from build123d import *

# Parameters (mm, degrees)
F0_W     = 38.1
F0_H     = 63.5
F1_DEPTH = 9.525
F2_W     = 38.1
F2_H     = 9.525
F3_DEPTH = 31.75
F4_R     = 8.75
F5_DEPTH = 6.35
F6_R     = 6.35
F7_DEPTH = 25.4
F4_R_2   = 8.7503
F8_DEPTH = 6.35


with BuildPart() as f1:
    # F0 (on Top) → F1 (new body)
    with BuildSketch(Plane.XY):
        with Locations((19.05, 31.75)):
            Rectangle(F0_W, F0_H)
    extrude(amount=F1_DEPTH)

    # F2 (on face) → F3 (join)
    with BuildSketch(Plane.XY.offset(9.525)):
        with Locations((19.05, 4.7625)):
            Rectangle(F2_W, F2_H)
    extrude(amount=F3_DEPTH)

    # F4 (on face) → F5 (cut)
    with BuildSketch(Plane(origin=(0, 0, 0), x_dir=(1, 0, 0), z_dir=(0, 0, -1))):
        with Locations((19.05, -44.45)):
            Circle(F4_R)
    extrude(amount=-F5_DEPTH, mode=Mode.SUBTRACT)

    # F6 (on face) → F7 (cut)
    with BuildSketch(Plane(origin=(0, 9.525, 0), x_dir=(-1, 0, 0), z_dir=(0, 1, 0))):
        with Locations((-19.05, 28.575)):
            Circle(F6_R)
    extrude(amount=-F7_DEPTH, mode=Mode.SUBTRACT)

    # F4 (on face) → F8 (cut)
    with BuildSketch(Plane(origin=(0, 0, 0), x_dir=(1, 0, 0), z_dir=(0, 0, -1))):
        with Locations((19.05, -44.45)):
            Circle(F4_R)
        with Locations((19.05, -12.7)):
            Circle(F4_R_2)
    extrude(amount=-F8_DEPTH, mode=Mode.SUBTRACT)


solid = f1.part
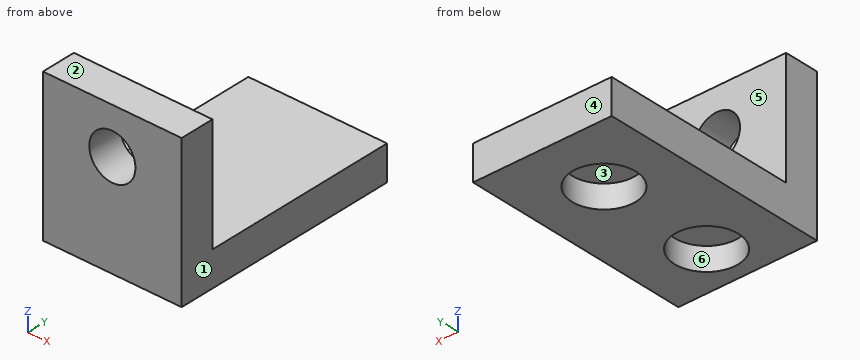
Check sheet for the modelled part. Datum: model origin and axes. Units: mm. Face numbers are marked on the shaded views. A direction names the side the tool comes from. Coordinates: 2 decimals unless noted, no trailing zeros. Loops run counter-clockwise (first coordinate to the right, second up) from the corner with the lowest first, then second, coordinate; pieces in that order, holes last. Notation, with made-up numbers: (40.5, 66.25) -> (65.5, 66.25) arc R14 ccw to (65.5, 70.25) -> close; hole circle Ø1 at (80.5, 73.25). An arc over 180 degrees is marked (long way). Write item = value, one per line. Start each with the question number.
1. Section check B-B on y = 44.45. Record the cut outline in (x, z) (3 decimals), then the cut area to 3 significant figures.
2. Section check D-D on z = 33.5. Record the cut outline in (x, y) (3 decimals).
3. Tool access check on the marked faces 4, 5 and 6. Record the directions out of +Z, -Z, +X, -X, +Y, -Y that give a thin tool (end or side, any length) a straight path to the whole face; none if there is none.
4. Section check A-A on x = 19.05. Record the cut outline in (y, z) (3 decimals), then the cut area to 3 significant figures.
5. Depth check by flat-ended pin: P1, Ø16, axis at x = 19.05, y = 12.7, coming from the -Z side; P2, Ø1, axis at x = 4.5, z = 28, coming from the -Y side; P3, Ø4, axis at x = 19.5, y = 19, coming from the +Z side (3 decimals); P4, Ø16, axis at x = 16.5, z = 27.5, coming from the +Y side (3 decimals). Enter the tip coordinate at first touch or a pass-through.
6. Material ranges on line 1 (Y direction, x = 19.05, z = 5); line 2 (Y direction, x = 2.5, z = 33.5) (3 decimals); line 3 (Z direction, x = 19, y = 2) (3 decimals), recorded low to high.
7. Section check C-C on y = 7.5. Record the cut outline in (x, z) (3 decimals).
8. Draft check along X on the marked faces 1, 2 and 3. Enter one of: released by +X, released by -X, zero draft, split by the parting line, or undercut.
Responses:
q1.outline = (0, 0) -> (10.3, 0) -> (10.3, 6.35) -> (27.8, 6.35) -> (27.8, 0) -> (38.1, 0) -> (38.1, 9.525) -> (0, 9.525) -> close
q1.area = 252 mm2
q2.outline = (0, 0) -> (15.042, 0) -> (15.042, 9.525) -> (0, 9.525) -> close; (23.058, 0) -> (38.1, 0) -> (38.1, 9.525) -> (23.058, 9.525) -> close
q3.face_4 = +Z, -Z, +X, -X, +Y
q3.face_5 = +Z, +X, -X, +Y
q3.face_6 = -Z
q4.outline = (0, 0) -> (3.95, 0) -> (3.95, 6.35) -> (21.45, 6.35) -> (21.45, 0) -> (35.7, 0) -> (35.7, 6.35) -> (53.2, 6.35) -> (53.2, 0) -> (63.5, 0) -> (63.5, 9.525) -> (9.525, 9.525) -> (9.525, 22.225) -> (0, 22.225) -> close; (0, 34.925) -> (9.525, 34.925) -> (9.525, 41.275) -> (0, 41.275) -> close
q4.area = 564 mm2
q5.P1 = 6.35
q5.P2 = 0
q5.P3 = 9.525
q5.P4 = 9.525
q6.line_1 = 0 to 3.95, 21.45 to 35.7, 53.2 to 63.5
q6.line_2 = 0 to 9.525
q6.line_3 = 0 to 22.225, 34.925 to 41.275
q7.outline = (0, 0) -> (12.012, 0) -> (12.012, 6.35) -> (26.088, 6.35) -> (26.088, 0) -> (38.1, 0) -> (38.1, 41.275) -> (0, 41.275) -> close; hole circle Ø12.7 at (19.05, 28.575)
q8.face_1 = released by +X
q8.face_2 = zero draft
q8.face_3 = undercut
